Work out the finished part from the listing and answer in its coordinate system (mm). A direction names the side the tool comes from. Coordinates: 2 decimals unless noted, no trailing zeros. Write each loop counter-clockwise with the first axis right and the second up, starting at its lowest first coordinate (ties: lowest second). Pieces come first, ordered by that corner, then holes. Notation, with made-up numbers: (-11.75, -13) - (29.25, -13) arc R21 ccw to (29.25, 24) - close; hole circle Ø8 at (56, 1.25). An arc over 180 degrees is marked (long way). Use a Markdown table: item, result. Add a question column.
(1) The part is cut by section C-C, the plane x = 4.5. Give the vertices of the cut face in (y, z).
(2) Given pin 1 Ø2 at (x, z) = (34.5, 6.5) entering from -Y; pin 2 Ø5 at (y, z) = (18.5, 6.5) entering from +X; pin 3 Ø3 at (x, y) = (-61, 0.5) entering from -Z, each flat-ended and moving along its own axis, determine where each tip first touches the part or whether it passes through.
(3) For a pull along X with two mould halves and no side action, classify faces 1 (the face through (-78.497, 0.68, 6.162)), 2 (the face through (49.24, -49.55, 6.16)), 3 (the face through (0.68, 78.497, 6.162)), 4 (the face through (51, 1, 0)) as released by +X, released by -X, zero draft, split by the parting line, or undercut.
(4) The part is cut by section B-B, the plane y = 41.5. Give the vertices of the cut face in (x, z).
(5) The part is cut by section A-A, the plane z = 6.25. Give the vertices of the cut face in (x, y).
(6) The part is cut by section D-D, the plane y = 60. Give the vertices of the cut face in (x, z), then the cut area to 4 significant figures.
(7) A tool of negligible diameter and unlimited length cuts with its end or side. For faces 5 (the face through (-67, 0, 2)), 6 (the face through (51, 1, 12.5)), from which of +Z, -Z, +X, -X, +Y, -Y can it reach the whole face along a straight path? Write none if from no direction.
(8) Find the intervals of material crossed by line 1 (X direction, y = 4, z = 2.5); line 2 (Y direction, x = -62, z = 11.5); line 3 (X direction, y = -30.5, z = 0.5), in increasing order. Write a range as from..to.
from build123d import *

# Parameters (mm, degrees)
SKETCH_1_R          = 50
SKETCH_1_R_2        = 1.75
EXTRUDE_1_DEPTH     = 12.5
SKETCH_1_3_R        = 5
CUT_EXTRUDE_1_DEPTH = 4


with BuildPart() as part:
    # Sketch 1 → Extrude 1 (new body)
    with BuildSketch(Plane.XY):
        with BuildLine():
            ThreePointArc((63.94815926, -45.528924074), (78.5, 0), (63.94815926, 45.528924074))
            ThreePointArc((63.94815926, 45.528924074), (49.393398282, 49.393398282), (45.528924074, 63.94815926))
            ThreePointArc((45.528924074, 63.94815926), (0, 78.5), (-45.528924074, 63.94815926))
            ThreePointArc((-45.528924074, 63.94815926), (-49.393398282, 49.393398282), (-63.94815926, 45.528924074))
            ThreePointArc((-63.94815926, 45.528924074), (-78.5, 0), (-63.94815926, -45.528924074))
            ThreePointArc((-63.94815926, -45.528924074), (-49.393398282, -49.393398282), (-45.528924074, -63.94815926))
            ThreePointArc((-45.528924074, -63.94815926), (0, -78.5), (45.528924074, -63.94815926))
            ThreePointArc((45.528924074, -63.94815926), (49.393398282, -49.393398282), (63.94815926, -45.528924074))
        make_face()
        Circle(SKETCH_1_R, mode=Mode.SUBTRACT)
        with Locations((-62, 0)):
            Circle(SKETCH_1_R_2, mode=Mode.SUBTRACT)
        with Locations((62, 0)):
            Circle(SKETCH_1_R_2, mode=Mode.SUBTRACT)
    extrude(amount=EXTRUDE_1_DEPTH)

    # Sketch 1_3 → Cut-Extrude 1 (cut)
    with BuildSketch(Plane.XY):
        with Locations((-62, 0)):
            Circle(SKETCH_1_3_R)
        with Locations((62, 0)):
            Circle(SKETCH_1_3_R)
    extrude(amount=CUT_EXTRUDE_1_DEPTH, mode=Mode.SUBTRACT)


solid = part.part
Model answer:
| question | item | result |
|---|---|---|
| 1 | outline | (-78.37, 0) - (-49.8, 0) - (-49.8, 12.5) - (-78.37, 12.5) - close; (49.8, 0) - (78.37, 0) - (78.37, 12.5) - (49.8, 12.5) - close |
| 2 | pin 1 | y = -70.99 |
| 2 | pin 2 | x = 76.85 |
| 2 | pin 3 | z = 4 |
| 3 | face 1 | released by -X |
| 3 | face 2 | undercut |
| 3 | face 3 | split by the parting line |
| 3 | face 4 | zero draft |
| 4 | outline | (-66.63, 0) - (-27.89, 0) - (-27.89, 12.5) - (-66.63, 12.5) - close; (27.89, 0) - (66.63, 0) - (66.63, 12.5) - (27.89, 12.5) - close |
| 5 | outline | (-63.95, -45.53) arc R15 cw to (-45.53, -63.95) arc R78.5 ccw to (45.53, -63.95) arc R15 cw to (63.95, -45.53) arc R78.5 ccw to (63.95, 45.53) arc R15 cw to (45.53, 63.95) arc R78.5 ccw to (-45.53, 63.95) arc R15 cw to (-63.95, 45.53) arc R78.5 ccw to start; hole circle Ø3.5 at (-62, 0); hole circle Ø100 at (0, 0); hole circle Ø3.5 at (62, 0) |
| 6 | outline | (-45, 0) - (45, 0) - (45, 12.5) - (-45, 12.5) - close |
| 6 | area | 1,125 mm^2 |
| 7 | face 5 | -Z |
| 7 | face 6 | +Z, +X, -X, +Y, -Y |
| 8 | line 1 | -78.4..-65, -59..-49.84, 49.84..59, 65..78.4 |
| 8 | line 2 | -45.13..-1.75, 1.75..45.13 |
| 8 | line 3 | -72.33..-39.62, 39.62..72.33 |
